Geometry: final body of the model. Coordinates: model frame, mm. A direction names the side the tool comes from. Give positions to 0.01 mm unless a question says otherwise; leave off trailing zeros. Order: outer loops, then holes, each group sorted by start corner. A loop starts at its lowest first (then second) coordinate and runs counter-clockwise, first axis right, second up. Notation, with made-up numbers: (80.25, 43.25) - (133.25, 43.25) arc R13 ccw to (133.25, 67.25) - close; hole circle Ø7 at (29, 20). An arc over 180 degrees is marked (long way). Use one line per item in the form item = value.
from build123d import *


with BuildPart() as part:
    # Sketch1 → Revolve1 (revolve)
    with BuildSketch(Plane.XY, mode=Mode.PRIVATE) as revolve1_sk:
        with BuildLine():
            Line((22, 45), (-22, 45))
            Line((-22, 45), (-22, 50))
            Line((-22, 50), (-17, 50))
            Line((-17, 50), (-17, 49.99))
            ThreePointArc((-17, 49.99), (-16.270695885, 48.229304115), (-14.51, 47.5))
            Line((-14.51, 47.5), (14.51, 47.5))
            ThreePointArc((14.51, 47.5), (16.270695885, 48.229304115), (17, 49.99))
            Line((17, 49.99), (17, 50))
            Line((17, 50), (22, 50))
            Line((22, 50), (22, 45))
        make_face()
    revolve(revolve1_sk.sketch.rotate(Axis((62.978723404, 0, 0), (-1, 0, 0)), 90), axis=Axis((62.978723404, 0, 0), (-1, 0, 0)))


solid = part.part
(1) Pull-direction query (Z, two-part tool) for faces 3 (the face through (19.54, -15.02, -47.69)), 4 (the face through (-22, -19, -41)), 5 (the face through (-0.308, 39.923, -20.765)); classes: released by +Z, released by -Z, zero draft, split by the parting line, or undercut.
Computed values:
face_3 = split by the parting line
face_4 = zero draft
face_5 = undercut
(2) Cut plane B-B on x = 2. Output: boundary loops of the cut face in (y, z), plus the area to 3 significant figures.
Computed values:
outline = circle Ø95 at (0, 0); hole circle Ø90 at (0, 0)
area = 726 mm²
(3) Ray query, line 1 along Y through (x, z) = (3, 0); line 2 along Z through (x, y) = (6, -14.5); line 3 along Z through (x, y) = (15, -41). Return the intervals inside material, ascending.
Computed values:
line_1 = -47.5 to -45, 45 to 47.5
line_2 = -45.23 to -42.6, 42.6 to 45.23
line_3 = -24.08 to -18.55, 18.55 to 24.08
(4) Contact query for flat-ended pins moving along their axis: pin 1 Ø1 at (x, z) = (-11.5, 8) entering from -Y; pin 2 Ø10 at (x, z) = (10.5, 12) entering from +Y; pin 3 Ø8 at (x, y) = (10.5, -13.5) entering from +Z; pin 4 Ø4 at (y, z) = (-32, 39.5) entering from -X. Output: stop coordinate, or through.
Computed values:
pin_1 = -46.9
pin_2 = 46.98
pin_3 = 46.54
pin_4 = -22
(5) Reachability of faces 1 (the face through (0.2, 46.37, 10.3)), 2 (the face through (22, -19, 41)) from +Z, -Z, +X, -X, +Y, -Y: full face, straight path, thin tool, end or side. Return the list, or none.
Computed values:
face_1 = none
face_2 = +Z, -Z, +X, +Y, -Y
